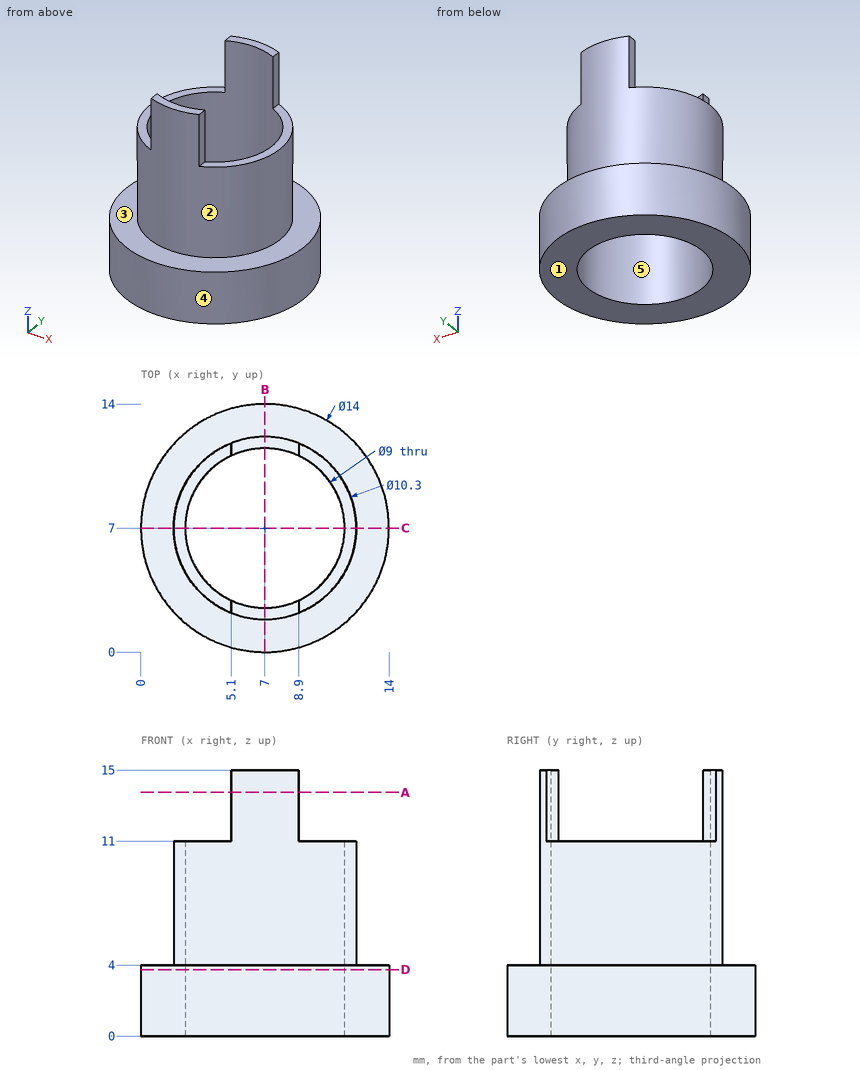
Drawing for the job (mm, zero at the part's lowest x, y, z). A direction names the side the tool comes from. Round coordinates to 2 decimals unless told otherwise and drop trailing zeros. Loops run counter-clockwise (first coordinate to the right, second up) from the corner with the lowest first, then second, coordinate; pieces in that order, holes last.
1. Mould opens along Y. For the marked faces 3, 4 and 5 say: +Y half, -Y half, draft (parallel to the pull), parting line (faces both ways), or undercut.
Check values:
face 3: draft
face 4: parting line
face 5: undercut
2. Drop flat-ended pins along their axis: P1, Ø1, axis at x = 10, y = 5.5, coming from the +Z side; P2, Ø0.8, axis at y = 2.5, z = 12.5, coming from the -X side; P3, Ø1.5, axis at x = 6, z = 8.5, coming from the +Y side; P4, Ø0.8, axis at y = 11.5, z = 12.5, coming from the +X side. Give the stop position or say it passes through.
Check values:
P1: passes through
P2: stops at x = 5.1
P3: stops at y = 12.14
P4: stops at x = 8.9
3. Band-saw the part on A-A, the plane z = 13.75. List the corners of the cut face in (x, y).
Check values:
outline: (5.1, 2.21) arc R5.15 ccw to (8.9, 2.21) - (8.9, 2.92) arc R4.5 cw to (5.1, 2.92) - close; (5.1, 11.08) arc R4.5 cw to (8.9, 11.08) - (8.9, 11.79) arc R5.15 ccw to (5.1, 11.79) - close
4. Band-saw the part on C-C, the plane y = 7. List the corners of the cut face in (x, z), and give its area (3 significant figures).
Check values:
outline: (0, 0) - (2.5, 0) - (2.5, 11) - (1.85, 11) - (1.85, 4) - (0, 4) - close; (11.5, 0) - (14, 0) - (14, 4) - (12.15, 4) - (12.15, 11) - (11.5, 11) - close
area: 29.1 mm2
5. Tool access for the marked faces 1 and 2: list every direction of +Z, -Z, +X, -X, +Y, -Y with a clear straight run to the whole face (end or side of a thin tool).
Check values:
face 1: -Z, +X, -X, +Y, -Y
face 2: +Z
6. Wall check: probe 1 along Y at (x, z) = (7, 8.25); probe 2 along Z at (x, y) = (12.5, 7.25). Give the ranges that are in metal, low to high.
Check values:
probe 1: y = 1.85 to 2.5, 11.5 to 12.15
probe 2: z = 0 to 4
7. Band-saw the part on D-D, the plane z = 3.75. List the corners of the cut face in (x, y).
Check values:
outline: circle Ø14 at (7, 7); hole circle Ø9 at (7, 7)
8. Band-saw the part on B-B, the plane x = 7. List the corners of the cut face in (y, z), and give its area (3 significant figures).
Check values:
outline: (0, 0) - (2.5, 0) - (2.5, 15) - (1.85, 15) - (1.85, 4) - (0, 4) - close; (11.5, 0) - (14, 0) - (14, 4) - (12.15, 4) - (12.15, 15) - (11.5, 15) - close
area: 34.3 mm2
